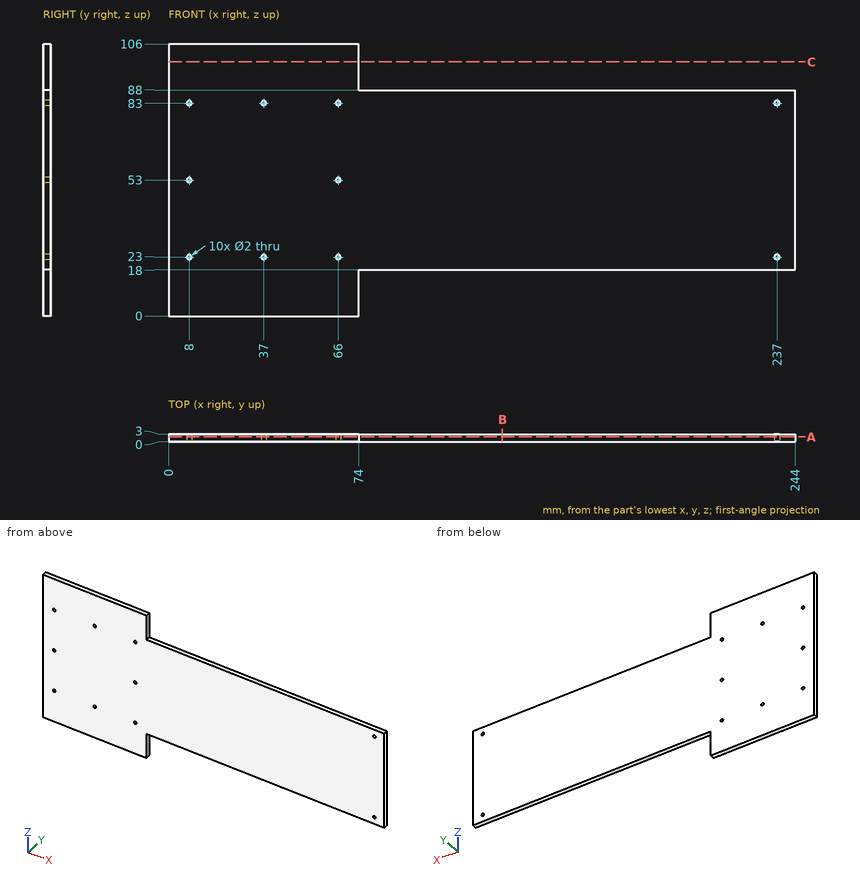
Part print with two shaded views. Sizes in mm from the minimum x, y, z corner. Round coordinates to 2 decimals unless told otherwise and drop trailing zeros. Write each loop counter-clockwise with the first axis right and the second up, starting at its lowest first coordinate (ties: lowest second). Pieces come first, ordered by that corner, then holes. Notation, with made-up numbers: M 40.25,-11 L 91.25,-11 A23 ccw 91.25,10 Z; hole C 35.25,14.5 d3. An arc over 180 degrees is marked long. Answer as CSV lines item,"result". Start each with the question number.
1) Drop flat-ended pins along their axis: pin 1 (0.9 mm diameter, centred on y = 1.5, z = 95.5, fed in from +X); pin 2 (0.9 mm diameter, centred on x = 185, y = 1, fed in from +Z). Give the stop position or say it passes through.
2) Band-saw the part on A-A (y = 1.9). Count the separate pieces of the cut face and the enclosed holes in it, then the cut area to 3 significant figures.
3) Drill centre lines: L1, parallel to Z at x = 66, y = 1.95; L2, parallel to Z at x = 237, y = 1.3; L3, parallel to X at y = 0.9, z = 53. Where is each one in solid material? Low to high.
4) Band-saw the part on B-B (x = 130). List the corners of the cut face in (y, z), then the cut area to 3 significant figures.
5) Band-saw the part on C-C (z = 99). List the corners of the cut face in (x, y), then the cut area to 3 significant figures.
Worked out:
1,pin 1,"x = 74"
1,pin 2,"z = 88"
2,separate pieces,"1"
2,enclosed holes,"10"
2,area,"19,700 mm²"
3,L1,"0 to 22, 24 to 52, 54 to 82, 84 to 106"
3,L2,"18 to 22, 24 to 82, 84 to 88"
3,L3,"0 to 7, 9 to 65, 67 to 244"
4,outline,"M 0,18 L 3,18 L 3,88 L 0,88 Z"
4,area,"210 mm²"
5,outline,"M 0,0 L 74,0 L 74,3 L 0,3 Z"
5,area,"222 mm²"
